```python
from build123d import *

# Parameters (mm, degrees)
F0_R     = 7
F1_DEPTH = 44
F2_W     = 34
F2_H     = 19
F3_DEPTH = 51.001
F4_W     = 35.544027
F4_H     = 19
F5_DEPTH = 19
F6_R     = 5.5
F7_DEPTH = 44.001


with BuildPart() as f1:
    # F0 (on Front) → F1 (new body)
    with BuildSketch(Plane.XZ):
        Polygon((-7, 18), (-14, 11), (-14, -7), (-7, -14), (20, -14), (20, 14.47346), (0, 18), align=None)
        Circle(F0_R, mode=Mode.SUBTRACT)
        with BuildLine():
            Line((22.361381, 14.057085), (20, 14.47346))
            Line((20, 14.47346), (20, -14))
            Line((20, -14), (25.575539, -14))
            ThreePointArc((25.575539, -14), (28.840775, -15.213414), (30.521178, -18.264706))
            ThreePointArc((30.521178, -18.264706), (32.858008, -26.115672), (37.29698, -33))
            Line((37.29698, -33), (43, -33))
            Line((43, -33), (72, 1))
            Line((72, 1), (72, 20))
            Line((72, 20), (67, 25))
            Line((67, 25), (43, 25))
            ThreePointArc((43, 25), (34.561099, 15.982044), (22.361381, 14.057085))
        make_face()
    extrude(amount=F1_DEPTH)

    # F2 (on face) → F3 (cut, through all)
    with BuildSketch(Plane.XY.offset(18)):
        with Locations((2.657733, -34.5)):
            Rectangle(F2_W, F2_H)
    extrude(amount=-F3_DEPTH, mode=Mode.SUBTRACT)

    # F4 (on face) → F5 (cut)
    with BuildSketch(Plane.XZ.offset(44)):
        with Locations((43.347552, -23.5)):
            Rectangle(F4_W, F4_H)
    extrude(amount=-F5_DEPTH, mode=Mode.SUBTRACT)

    # F6 (on face) → F7 (cut, through all)
    with BuildSketch(Plane.XZ.offset(44)):
        with Locations((58, 11.325206)):
            Circle(F6_R)
    extrude(amount=-F7_DEPTH, mode=Mode.SUBTRACT)


solid = f1.part
```
Geometry check sheet. Reference: the model listing, model coordinates, mm. A direction names the side the tool comes from. Give positions to 0.01 mm unless a question says otherwise; leave off trailing zeros. Loops run counter-clockwise (first coordinate to the right, second up) from the corner with the lowest first, then second, coordinate; pieces in that order, holes last. Notation, with made-up numbers: M 73,-6.75 L 117,-6.75 A28 cw 117,13.25 Z; hole C 49,-18.5 d5. An arc over 180 degrees is marked long. Answer as CSV lines item,"result".
Item 1: Cross-section at D-D on y = -10.5. Record the cut outline in (x, z), and give its area (3 significant figures).
Values:
outline,"M -14,-7 L -7,-14 L 25.58,-14 A5 cw 30.52,-18.26 A29 ccw 37.3,-33 L 43,-33 L 72,1 L 72,20 L 67,25 L 43,25 A19 cw 22.36,14.06 L 0,18 L -7,18 L -14,11 Z; hole C 0,0 d14; hole C 58,11.33 d11"
area,"2,830 mm²"
Item 2: Material ranges on line 1 (Z direction, x = 0, y = -8); line 2 (Y direction, x = 15, z = 6); line 3 (X direction, y = -11.5, z = 0), recorded low to high.
Values:
line 1,"z = -14 to -7, 7 to 18"
line 2,"y = -25 to 0"
line 3,"x = -14 to -7, 7 to 71.15"
Item 3: Cross-section at A-A on x = -6. Record the cut outline in (y, z).
Values:
outline,"M -25,-14 L 0,-14 L 0,-3.61 L -25,-3.61 Z; M -25,3.61 L 0,3.61 L 0,18 L -25,18 Z"
Item 4: Release check for a two-part mould opening along X. For faces 4 (the cylindrical face through (34.716, -21.692, 16.065)), 5 (the flat face through (-11, -12, -10)), 6 (the flat face through (70, -22, 22)) record: pulls with the +X half, pulls with the -X half, needs draft (parallel to the pull), parting line crosses it, or undercut.
Values:
face 4,"undercut"
face 5,"pulls with the -X half"
face 6,"pulls with the +X half"
Item 5: Cross-section at C-C on y = -37. Record the cut outline in (x, z), and give its area (3 significant figures).
Values:
outline,"M 19.66,-14 L 59.21,-14 L 72,1 L 72,20 L 67,25 L 43,25 A19 cw 22.36,14.06 L 19.66,14.53 Z; hole C 58,11.33 d11"
area,"1,630 mm²"
Item 6: Cross-section at B-B on z = 0. Record the cut outline in (x, y), and give its area (3 significant figures).
Values:
outline,"M -14,-25 L -7,-25 L -7,0 L -14,0 Z; M 7,-25 L 19.66,-25 L 19.66,-44 L 71.15,-44 L 71.15,0 L 7,0 Z"
area,"2,760 mm²"
Item 7: Access from +Z, -Z, +X, -X, +Y, -Y to the whole of each face (thin tool, end or side, straight path). Record for faces 1 (the flat face through (-3, -12, 18)), 2 (the flat face through (6, -25, 6)), 3 (the flat face through (26, -27, -14)).
Values:
face 1,"+Z, -X, +Y, -Y"
face 2,"+Z, -Z, -X, -Y"
face 3,"-Z, -X, -Y"
Item 8: Depth check by flat-ended pin: P1, Ø12, axis at x = 42, z = 9.5, coming from the +Y side; P2, Ø5, axis at y = -10.5, z = -13, coming from the -X side; P3, Ø6.5, axis at x = 58, z = 11.33, coming from the -Y side; P4, Ø1.5, axis at x = 39.5, y = -35, coming from the -Z side. Enter the tip coordinate at first touch or a pass-through.
Values:
P1,"stops at y = 0"
P2,"stops at x = -10.5"
P3,"passes through"
P4,"stops at z = -14"
